Source: three-view drawing plus pictorial views. Frame: mm from the lowest corner of the part. A direction names the side the tool comes from. Give positions to 0.01 mm unless a question says otherwise; leave off trailing zeros. Order: outer loops, then holes, each group sorted by start corner. A loop starts at its lowest first (then second) coordinate and runs counter-clockwise, first axis right, second up. Notation, with made-up numbers: (-39, 6.5) -> (-10, 6.5) arc R18 ccw to (-10, 27.5) -> close; hole circle Ø3 at (2.25, 82.5). An arc over 180 degrees is marked (long way). Use a Markdown table: item, result. Add a question column.
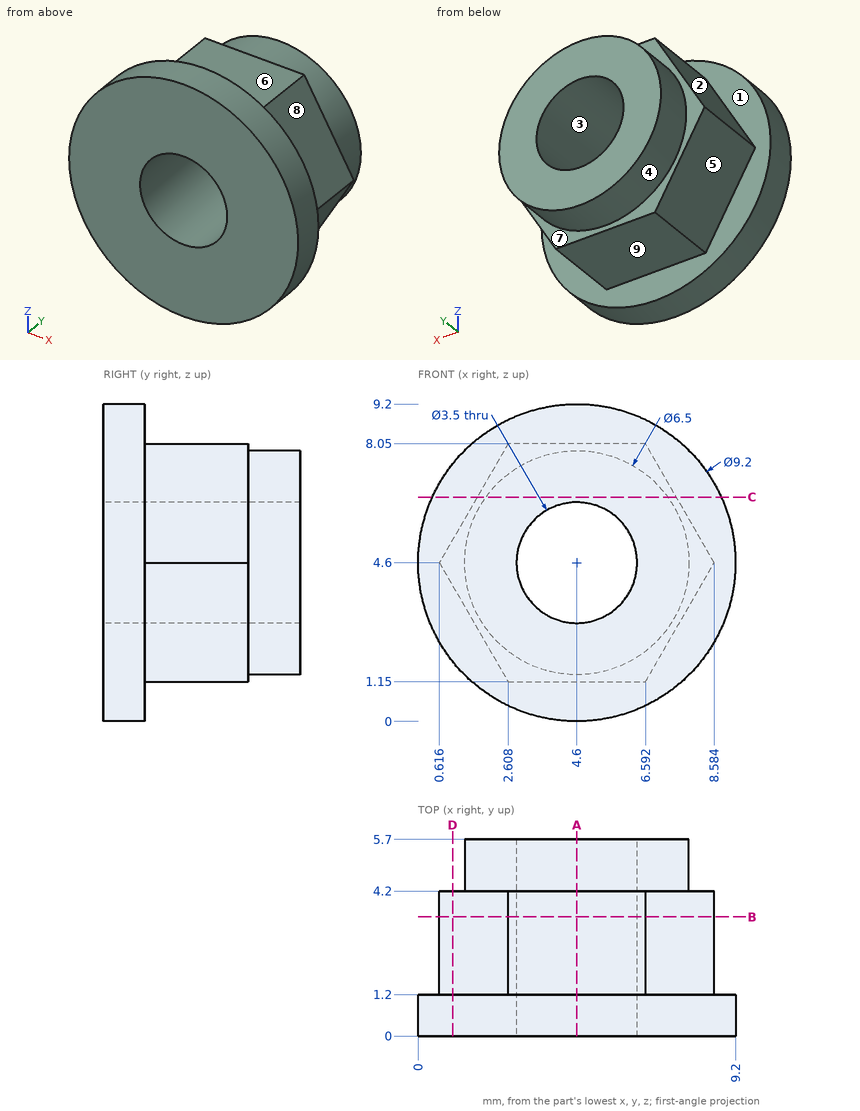
Q1. Access query for the marked faces 5, 6, 7, 8 and 9. Directions: +Z, -Z, +X, -X, +Y, -Y. A direction counts if a zero-diameter tool reaches every point of the face in a straight line with its end or side. Return the directions, or none.
Q2. Section query D-D (x = 1). Return loops of the section in (y, z) (1 decimal).
Q3. First-contact query: pin 1 (0.9 mm diameter, centred on x = 3.5, y = 3, fed in from +Z); pin 2 (1.5 mm diameter, centred on x = 3, y = 0.5, fed in from -Z); pin 3 (3 mm diameter, centred on y = 2.5, z = 7, fed in from -X). Flat tips, straight axial feed; report the tip coordinate or a pass-through.
Q4. Section query B-B (y = 3.45). Return loops of the section in (x, z), plus the area to 3 significant figures.
Q5. Section query A-A (x = 4.6). Return loops of the section in (y, z).
Q6. Ray query, line 1 (Z direction, x = 4.6, y = 3); line 2 (Y direction, x = 8.75, z = 5.25); line 3 (Y direction, x = 1.75, z = 2.75). Return the intervals inside material, ascending.
Q7. Section query C-C (z = 6.5). Return loops of the section in (x, y).
Q8. Draft query along X for the marked faces 1, 2, 3 and 4. Return one class per face: +X half, -X half, draft (parallel to the pull), parting line (faces both ways), or undercut.
Solution:
| question | item | result |
|---|---|---|
| 1 | face 5 | -Z, -X, +Y |
| 1 | face 6 | +Z, +X, -X, +Y |
| 1 | face 7 | +Y |
| 1 | face 8 | +Z, +X, +Y |
| 1 | face 9 | -Z, +X, -X, +Y |
| 2 | outline | (0, 1.7) -> (1.2, 1.7) -> (1.2, 3.9) -> (4.2, 3.9) -> (4.2, 5.3) -> (1.2, 5.3) -> (1.2, 7.5) -> (0, 7.5) -> close |
| 3 | pin 1 | stops at z = 8.05 |
| 3 | pin 2 | stops at z = 0.08 |
| 3 | pin 3 | stops at x = 0.31 |
| 4 | outline | (0.62, 4.6) -> (2.61, 1.15) -> (6.59, 1.15) -> (8.58, 4.6) -> (6.59, 8.05) -> (2.61, 8.05) -> close; hole circle Ø3.5 at (4.6, 4.6) |
| 4 | area | 31.6 mm² |
| 5 | outline | (0, 0) -> (1.2, 0) -> (1.2, 1.15) -> (4.2, 1.15) -> (4.2, 1.35) -> (5.7, 1.35) -> (5.7, 2.85) -> (0, 2.85) -> close; (0, 6.35) -> (5.7, 6.35) -> (5.7, 7.85) -> (4.2, 7.85) -> (4.2, 8.05) -> (1.2, 8.05) -> (1.2, 9.2) -> (0, 9.2) -> close |
| 6 | line 1 | z = 1.15 to 2.85, 6.35 to 8.05 |
| 6 | line 2 | y = 0 to 1.2 |
| 6 | line 3 | y = 0 to 4.2 |
| 7 | outline | (0.41, 0) -> (8.79, 0) -> (8.79, 1.2) -> (7.49, 1.2) -> (7.49, 4.2) -> (7.24, 4.2) -> (7.24, 5.7) -> (1.96, 5.7) -> (1.96, 4.2) -> (1.71, 4.2) -> (1.71, 1.2) -> (0.41, 1.2) -> close |
| 8 | face 1 | draft |
| 8 | face 2 | -X half |
| 8 | face 3 | undercut |
| 8 | face 4 | parting line |
